For this review, take the finished solid that the model builds, in its own axes (mm). A direction names the side the tool comes from. Round coordinates to 2 decimals unless told otherwise and drop trailing zeros. Write each loop counter-clockwise with the first axis right and the second up, starting at its lowest first coordinate (ties: lowest second). Pieces come first, ordered by that corner, then holes. Notation, with made-up numbers: M 61,48.5 L 100,48.5 A15 cw 100,71.5 Z; hole C 34,83 d6. An arc over 180 degrees is marked long. One line per question, with ' | ' between items.
```python
from build123d import *

# Parameters (mm, degrees)
SKETCH_2_R          = 3
CUT_EXTRUDE_1_DEPTH = 10
SKETCH_3_R          = 2
CUT_EXTRUDE_2_DEPTH = 21
SKETCH_4_R          = 5.5
SKETCH_4_R_2        = 4
CUT_EXTRUDE_3_DEPTH = 5.5


with BuildPart() as part:
    # Эскиз1 → Повернуть1 (revolve)
    with BuildSketch(Plane.XY):
        Polygon((4, 20), (4, 11), (5.5, 11), (5.5, 0), (0, 0), (0, 20), align=None)
    revolve(axis=Axis((0, 0, 0), (0, 1, 0)))

    # Эскиз2 → Вырез-Вытянуть1 (cut)
    with BuildSketch(Plane(origin=(0, 20, 0), x_dir=(1, 0, 0), z_dir=(0, 1, 0))):
        Circle(SKETCH_2_R)
    extrude(amount=-CUT_EXTRUDE_1_DEPTH, mode=Mode.SUBTRACT)

    # Эскиз3 → Вырез-Вытянуть2 (cut, through all)
    with BuildSketch(Plane.XZ):
        Circle(SKETCH_3_R)
    extrude(amount=-CUT_EXTRUDE_2_DEPTH, mode=Mode.SUBTRACT)

    # Эскиз4 → Вырез-Вытянуть3 (cut)
    with BuildSketch(Plane(origin=(0, 11, 0), x_dir=(1, 0, 0), z_dir=(0, 1, 0))):
        Circle(SKETCH_4_R)
        Circle(SKETCH_4_R_2, mode=Mode.SUBTRACT)
    extrude(amount=-CUT_EXTRUDE_3_DEPTH, mode=Mode.SUBTRACT)


solid = part.part
```
Item 1: Take a section at A-A (x = 0). Write out the cut boundary in (y, z).
Results:
outline: M 0,-5.5 L 5.5,-5.5 L 5.5,-4 L 20,-4 L 20,-3 L 10,-3 L 10,-2 L 0,-2 Z; M 0,2 L 10,2 L 10,3 L 20,3 L 20,4 L 5.5,4 L 5.5,5.5 L 0,5.5 Z
Item 2: Take a section at D-D (y = 3.75). Write out the cut boundary in (x, z), then the cut area to 3 significant figures.
Results:
outline: C 0,0 d11; hole C 0,0 d4 | area: 82.5 mm2
Item 3: To check wall thickness, follow line 1 along X through (y, z) = (13, 0); line 2 along Z through (x, y) = (0, 7). State the ranges of each line that lie inside material, in increasing order. Write a range as from..to.
Results:
line 1: -4..-3, 3..4 | line 2: -4..-2, 2..4
Item 4: Machinability: for faces 1 (the face through (-1, 20, -3)), 2 (the face through (-3, 15, 0)), which of the approach directions +Z, -Z, +X, -X, +Y, -Y give a long, thin tool a straight path to every point of the face, cutting with its end or side? Answer none if there is none.
Results:
face 1: +Z, -Z, +X, -X, +Y | face 2: +Y
Item 5: Mouldability with a two-part tool opening along Z and no side actions: class faces 3 (the face through (0, 5, -2)), 4 (the face through (-0.1, 0, 2.4)), 5 (the face through (-1.19, 2.71, 5.37)) as +Z half, -Z half, draft (parallel to the pull), parting line (faces both ways), or undercut.
Results:
face 3: undercut | face 4: draft | face 5: parting line
Item 6: Take a section at C-C (y = 11.75). Write out the cut boundary in (x, z).
Results:
outline: C 0,0 d8; hole C 0,0 d6
Item 7: Take a section at B-B (z = 0). Write out the cut boundary in (x, y), then the cut area to 3 significant figures.
Results:
outline: M -5.5,0 L -2,0 L -2,10 L -3,10 L -3,20 L -4,20 L -4,5.5 L -5.5,5.5 Z; M 2,0 L 5.5,0 L 5.5,5.5 L 4,5.5 L 4,20 L 3,20 L 3,10 L 2,10 Z | area: 76.5 mm2
Item 8: Insertion check: pin 1 Ø5 at (x, y) = (-3, 9.5) entering from -Z; pin 2 Ø3 at (x, y) = (-3, 6.5) entering from +Z; pin 3 Ø6 at (y, z) = (11, -1) entering from -X. Each pin has a flat end and moves straight along its axis. Give the tip position at first contact, or say it passes through.
Results:
pin 1: z = -3.97 | pin 2: z = 5.17 | pin 3: x = -4
